Verification items for the finished model (mm, model axes). Face numbers are marked on the shaded views. A direction names the side the tool comes from. Round coordinates to 2 decimals unless told otherwise and drop trailing zeros. Write each loop counter-clockwise with the first axis right and the second up, starting at its lowest first coordinate (ties: lowest second). Pieces come first, ordered by that corner, then holes. Notation, with made-up numbers: M 38,88 L 42,88 A21 cw 42,98 Z; hole C -28.75,74 d9. An arc over 180 degrees is marked long. Write each question's results on one line, items separated by ' | '.
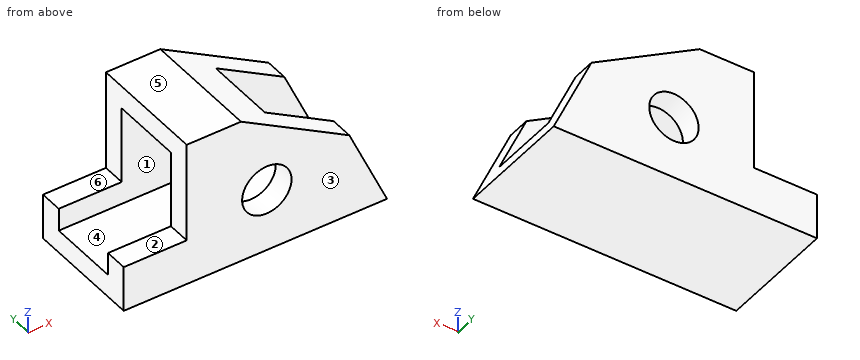
from build123d import *

# Parameters (mm, degrees)
F1_DEPTH = 41
F2_W     = 25
F2_H     = 35
F3_DEPTH = 92.001
F4_R     = 8.623428
F5_DEPTH = 41.001


with BuildPart() as f1:
    # F0 (on Front) → F1 (new body)
    with BuildSketch(Plane.XZ):
        Polygon((0, 16), (0, 0), (92, 0), (78.824782, 29.161852), (41, 51), (22, 51), (22, 16), align=None)
    extrude(amount=-F1_DEPTH)

    # F2 (on Right) → F3 (cut, through all)
    with BuildSketch(Plane.YZ):
        with Locations((20.5, 25.5)):
            Rectangle(F2_W, F2_H)
    extrude(amount=F3_DEPTH, mode=Mode.SUBTRACT)

    # F4 (on face) → F5 (cut, through all)
    with BuildSketch(Plane.XZ):
        with Locations((50, 22)):
            Circle(F4_R)
    extrude(amount=-F5_DEPTH, mode=Mode.SUBTRACT)


solid = f1.part
1) Depth check by flat-ended pin: P1, Ø4, axis at x = 65.5, z = 16, coming from the -Y side; P2, Ø20, axis at x = 60, y = 21.5, coming from the +Z side; P3, Ø9, axis at x = 10.5, y = 5, coming from the +Z side; P4, Ø10.5, axis at x = 50, z = 22, coming from the -Y side. Enter the tip coordinate at first touch or a pass-through.
Calculated:
P1: stops at y = 0 | P2: stops at z = 45.8 | P3: stops at z = 16 | P4: passes through
2) Access from +Z, -Z, +X, -X, +Y, -Y to the whole of each face (thin tool, end or side, straight path). Record for the marked faces 4, 5 and 6.
Calculated:
face 4: +X, -X | face 5: +Z, +X, -X, +Y, -Y | face 6: +Z, -X, +Y, -Y
3) Material ranges on line 1 (Y direction, x = 82, z = 18); line 2 (Z direction, x = 32, y = 14); line 3 (Z direction, x = 50, y = 6), recorded low to high. Write a range as [from, to].
Calculated:
line 1: y = [0, 8], [33, 41] | line 2: z = [0, 8], [43, 51] | line 3: z = [0, 13.38], [30.62, 45.8]
4) Sectioned sample at A-A, the plane y = 9. Record the cut outline in (x, z), and give its area (3 significant figures).
Calculated:
outline: M 0,0 L 92,0 L 88.39,8 L 0,8 Z; M 22,43 L 54.86,43 L 41,51 L 22,51 Z | area: 929 mm²
5) Sectioned sample at D-D, the plane z = 24. Record the cut outline in (x, y), and give its area (3 significant figures).
Calculated:
outline: M 22,0 L 41.61,0 L 41.61,8 L 22,8 Z; M 22,33 L 41.61,33 L 41.61,41 L 22,41 Z; M 58.39,0 L 81.16,0 L 81.16,8 L 58.39,8 Z; M 58.39,33 L 81.16,33 L 81.16,41 L 58.39,41 Z | area: 678 mm²
6) Draft check along Y on the marked faces 1, 2 and 3. Enter one of: pulls with the +Y half, pulls with the -Y half, needs draft (parallel to the pull), parting line crosses it, or undercut.
Calculated:
face 1: undercut | face 2: needs draft | face 3: pulls with the -Y half
7) Sectioned sample at C-C, the plane x = 46. Record the cut outline in (y, z).
Calculated:
outline: M 0,0 L 41,0 L 41,14.36 L 33,14.36 L 33,8 L 8,8 L 8,14.36 L 0,14.36 Z; M 0,29.64 L 8,29.64 L 8,43 L 33,43 L 33,29.64 L 41,29.64 L 41,48.11 L 0,48.11 Z
8) Sectioned sample at B-B, the plane z = 37.5. Record the cut outline in (x, y).
Calculated:
outline: M 22,0 L 64.38,0 L 64.38,8 L 22,8 Z; M 22,33 L 64.38,33 L 64.38,41 L 22,41 Z
